```python
from build123d import *

# Parameters (mm, degrees)
F0_W     = 40
F0_H     = 40
F1_DEPTH = 40
F4_R     = 5


with BuildPart() as f1:
    # F0 (on Top) → F1 (new body)
    with BuildSketch(Plane.XY):
        Rectangle(F0_W, F0_H)
    extrude(amount=F1_DEPTH)

    # F2 (on Front) → F3 (revolve, cut)
    with BuildSketch(Plane.XZ):
        with BuildLine():
            ThreePointArc((0, -4.756929), (24.378702, 20.243071), (0, 45.243071))
            Line((0, 45.243071), (0, -4.756929))
        make_face()
    revolve(axis=Axis((0, 0, 20.243071), (0, 0, -1)), mode=Mode.SUBTRACT)

    # F4
    f4_edges = [f1.edges().sort_by_distance(p)[0] for p in [
        (-20, 0, 40),
        (-20, -20, 20),
        (0, -20, 40),
        (0, -20, 0),
        (-20, 0, 0),
        (0, 20, 0),
        (-20, 20, 20),
        (20, 0, 0),
        (20, 20, 20),
        (20, -20, 20),
        (20, 0, 40),
        (0, 20, 40),
    ]]
    fillet(f4_edges, radius=F4_R)


solid = f1.part
```
Build history of the part. All positions in model axes, mm. Give positions to 0.01 mm unless a question says otherwise; leave off trailing zeros. One line per question, with ' | ' between items.
Q1. Drop a flat-ended pin along its axis: pin 1 (12 mm diameter, centred on x = 1.5, y = -5, fed in from +Z). Give the stop position or say it passes through.
Filled sheet:
pin 1: passes through
Q2. Drill centre lines: line 1 along Y through (x, z) = (13.5, 2.5); line 2 along Z through (x, y) = (-16, -0.5); line 3 along Z through (x, y) = (-11.5, 18). Where is each one in solid material? Low to high. Write a range as [from, to].
Filled sheet:
line 1: y = [-19.33, -10.32], [10.32, 19.33] | line 2: z = [0.1, 1.57], [38.91, 39.9] | line 3: z = [1, 8.33], [32.15, 39]
Q3. Cut at A-A, the plane x = 4. Count the separate pieces of the cut face and the enclosed holes in it, plus the area to 3 significant figures.
Filled sheet:
separate pieces: 4 | enclosed holes: 0 | area: 48.8 mm²
